Autodesk Inventor part; units mm, degrees
ref_plane "YZ Plane" through (0, 0, 0) normal (1, 0, 0) x (0, 1, 0)
ref_plane "XZ Plane" through (0, 0, 0) normal (0, 1, 0) x (-1, 0, 0)
ref_plane "XY Plane" through (0, 0, 0) normal (0, 0, 1) x (1, 0, 0)
sketch "Boceto1" plane through (0, 0, 0) normal (0, 1, 0) x (-1, 0, 0)
  circle A0 centre (0, 0) radius 2.5
  arc A1 (0, 10) -> (0, -10) centre (0, 0) ccw
  circle A2 centre (20.9, 0) radius 2.5
  arc A3 (20.9, -10) -> (20.9, 10) centre (20.9, 0) ccw
  line L0 (20.9, 10) -> (14.95, 10)
  line L1 (5.95, 10) -> (0, 10)
  line L2 (14.95, 10) -> (14.95, 24)
  line L3 (14.95, 24) -> (5.95, 24)
  line L4 (5.95, 24) -> (5.95, 10)
  line L5 (10.45, 9) -> (12.45, 9)
  line L6 (12.45, 9) -> (8.45, 9)
  circle A4 centre (10.45, 11.5) radius 1.5
  line L7 (12.45, 9) -> (14.95, 11.5)
  line L8 (8.45, 9) -> (5.95, 11.5)
  circle A5 centre (10.45, -11.5) radius 1.5
  arc A6 (8.0005, -12) -> (12.8995, -12) centre (10.45, -11.5) ccw
  line L9 (20.9, -10) -> (15.349, -10)
  line L10 (0, -10) -> (5.551, -10)
  arc A7 (8.0005, -12) -> (5.551, -10) centre (5.551, -12.5) ccw
  arc A8 (15.349, -10) -> (12.8995, -12) centre (15.349, -12.5) ccw
  circle A9 centre (10.45, -11.5) radius 2.5
  point P0 (8.45, -10)
  point P1 (12.45, -10)
  dimension "d10" = 5
  dimension "d11" = 20
  dimension "d13" = 5
  dimension "d14" = 20
  dimension "d19" = 9
  dimension "d20" = 14
  dimension "d25" = 3
  dimension "d27" = 3
  dimension "d28" = 5
  dimension "d29" = 2.5
  dimension "d30" = 5
extrude "Extrusión1" add sketch "Boceto1" along normal blind 6 contours A0 | L4 L3 L2 L7 L5 L6 L8 | A9 A6 | A2
extrude "Extrusión2" add sketch "Boceto1" along normal blind 2 contours L1 L4 L8 L6 L5 L7 L2 L0 A3 L9 A8 A9 A7 L10 A1
sketch "Boceto2" plane through (-5.95, 0, 24) normal (1, 0, 0) x (0, 0, -1)
  line L0 (0, 0) -> (14, 0)
  line L1 (14, 0) -> (14, 2)
  line L2 (12.5, 2) -> (14, 2)
  line L3 (12.5, 2) -> (12.5, 6)
  line L4 (0, 6) -> (12.5, 6)
  line L5 (0, 0) -> (0, 6)
  line L6 (0, 6) -> (12.5, 6)
  line L7 (0, 6) -> (0, 3)
  line L8 (0, 0) -> (0, 6)
  line L9 (0, 3) -> (3, 3)
  circle A0 centre (3, 3) radius 3
  circle A1 centre (3, 3) radius 1.75
  line L10 (0, 6) -> (3, 6)
  line L11 (0, 3) -> (0, 0)
  point P0 (24, 0)
  point P1 (3, 6)
  point P2 (3, 0)
  dimension "d37" = 6
  dimension "d35" = 3
  dimension "d36" = 3
  dimension "d38" = 3.5
extrude "Extrusión3" cut sketch "Boceto2" against normal blind 9 contours L5 A0 L0 | A1 | L5 L4 A0
properties part number "basedelapinza1"
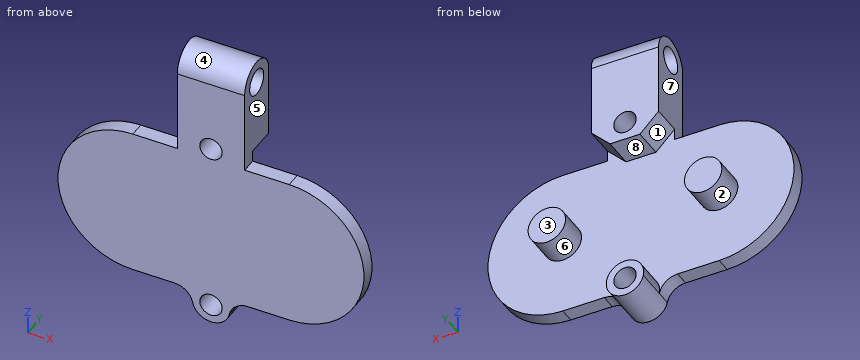
Work out the finished part from the listing and answer in its coordinate system (mm). Face numbers are marked on the shaded views. A direction names the side the tool comes from. Round coordinates to 2 decimals unless told otherwise and drop trailing zeros. Write each loop counter-clockwise with the first axis right and the second up, starting at its lowest first coordinate (ties: lowest second). Pieces come first, ordered by that corner, then holes. Notation, with made-up numbers: M 49.5,81 L 90.5,81 A25 ccw 90.5,104 Z; hole C 48,79 d10. An arc over 180 degrees is marked long. Use a Markdown table: item, result.
1) The part is cut by section B-B on y = 5.45. Give the vertices of the cut face in (x, z).
Taken from the geometry:
| item | result |
|---|---|
| outline | C -20.9,0 d5; M -14.95,11.5 L -12.45,9 L -8.45,9 L -5.95,11.5 L -5.95,22.73 L -14.95,22.73 Z; C -10.45,-11.5 d5; C 0,0 d5; hole C -10.45,-11.5 d3; hole C -10.45,11.5 d3 |
2) Consider line 1 (Z direction, x = -11.25, y = 3); line 2 (Z direction, x = -8.5, y = 3); line 3 (Y direction, x = -12, z = 21). Determine where each line is inside the solid, lowest interval first. Write a range as [from, to].
Taken from the geometry:
| item | result |
|---|---|
| line 1 | z = [-13.87, -12.77], [-10.23, -9.13], [9, 10.23], [12.77, 19.25], [22.75, 24] |
| line 2 | z = [-13.06, -9.94], [9, 19.25], [22.75, 24] |
| line 3 | y = [0, 1.25], [4.75, 6] |
3) The part is cut by section A-A on y = 3. Give the vertices of the cut face in (x, z).
Taken from the geometry:
| item | result |
|---|---|
| outline | C -20.9,0 d5; M -14.95,11.5 L -12.45,9 L -8.45,9 L -5.95,11.5 L -5.95,19.25 L -14.95,19.25 Z; M -14.95,22.75 L -5.95,22.75 L -5.95,24 L -14.95,24 Z; C -10.45,-11.5 d5; C 0,0 d5; hole C -10.45,-11.5 d3; hole C -10.45,11.5 d3 |
4) The part is cut by section D-D on y = 0.6. Give the vertices of the cut face in (x, z).
Taken from the geometry:
| item | result |
|---|---|
| outline | M -20.9,-10 L -15.35,-10 A2.5 cw -12.9,-12 A2.5 ccw -8,-12 A2.5 cw -5.55,-10 L 0,-10 A10 ccw 0,10 L -5.95,10 L -5.95,22.8 L -14.95,22.8 L -14.95,10 L -20.9,10 A10 ccw Z; hole C -10.45,-11.5 d3; hole C -10.45,11.5 d3 |
5) Which of the six approach directions +Z, -Z, +X, -X, +Y, -Y give full straight-line access (tool end or side, diameter ignored) to the marked faces 5, 6, 7 and 8?
Taken from the geometry:
| item | result |
|---|---|
| face 5 | +Z, +X, +Y, -Y |
| face 6 | +Y |
| face 7 | +Z, -X, +Y, -Y |
| face 8 | +X, -X, +Y |
6) Determine the mould class of the marked faces 1, 2, 3 and 4 for opening direction Z: pulls with the +Z half, pulls with the -Z half, needs draft (parallel to the pull), parting line crosses it, or undercut.
Taken from the geometry:
| item | result |
|---|---|
| face 1 | undercut |
| face 2 | parting line crosses it |
| face 3 | needs draft |
| face 4 | pulls with the +Z half |
7) Flat-ended cylindrical pins translate along their axes: pin 1 (2 mm diameter, centred on x = -18, y = 1, fed in from -Z); pin 2 (3 mm diameter, centred on y = 3, z = 21, fed in from +X); pin 3 (1 mm diameter, centred on x = -19, y = 1, fed in from +Z); pin 4 (3 mm diameter, centred on y = 2, z = 16, fed in from +X). Find the tip coordinate at first contact, or state that the pin passes through.
Taken from the geometry:
| item | result |
|---|---|
| pin 1 | stops at z = -10 |
| pin 2 | passes through |
| pin 3 | stops at z = 10 |
| pin 4 | stops at x = -5.95 |
8) The part is cut by section C-C on z = -11.5. Give the vertices of the cut face in (x, y).
Taken from the geometry:
| item | result |
|---|---|
| outline | M -13.06,0 L -11.95,0 L -11.95,6 L -12.95,6 L -12.95,2 L -13.06,2 Z; M -8.95,0 L -7.84,0 L -7.84,2 L -7.95,2 L -7.95,6 L -8.95,6 Z |
